The listing builds one solid part. Answer for the finished solid, in the listing's coordinates (mm). A direction names the side the tool comes from. Give positions to 0.01 mm unless a question says otherwise; leave off trailing zeros. Order: outer loops, then holes, each group sorted by start corner. A loop starts at its lowest first (then second) coordinate and runs counter-clockwise, first axis right, second up. Notation, with made-up numbers: (-4, 20) - (26, 20) arc R33 cw to (26, 54) - close; hole circle Ø6 at (79.25, -31.75). An arc over 180 degrees is marked (long way). Answer as a JSON object with one key per item and string values. Group by question number.
Q1. For faces 1 (the face through (91, 11, -11.5)), 2 (the face through (167.3, 15.2, -10)), 3 (the face through (151.831, 5.526, -13.021)), determine the directions among +Z, -Z, +X, -X, +Y, -Y from which every point of the face is accessible in a straight line to the end or side of a thin tool.
Q2. Consider line 1 (X direction, y = 13.25, z = 0); line 2 (X direction, y = 19, z = 5.5); line 3 (Y direction, x = 26.5, z = -13.25). Determine where each line is inside the solid, lowest interval first.
Q3. A cutting plane is placed at C-C, the plane y = 5. Give the vertices of the cut face in (x, z).
Q4. Given pin 1 (5.5 mm diameter, centred on x = 26.5, y = 5, fed in from +Z); pin 2 (4 mm diameter, centred on y = 13.5, z = 11, fed in from -X); pin 3 (8 mm diameter, centred on y = 9, z = 0.5, fed in from +X); pin 4 (1 mm diameter, centred on y = 13.5, z = 8, fed in from -X), each flat-ended and moving along its own axis, determine where each tip first touches the part or whether it passes through.
Q5. A cutting plane is placed at A-A, the plane x = 26.5. Give the vertices of the cut face in (y, z).
Q6. A cutting plane is placed at B-B, the plane z = 0. Give the vertices of the cut face in (x, y).
Q7. A cutting plane is placed at D-D, the plane y = 20.5. Count the separate pieces of the cut face and the enclosed holes in it, and give its area (3 significant figures).
Q8. The mould has two halves that part along Z. Classify faces 4 (the face through (98, 0, -12)), 5 (the face through (189.7, 14.79, 6.18)), 6 (the face through (89, 11, -14.5)), 7 (the face through (12.7, 15.2, -10)): released by +Z, released by -Z, zero draft, split by the parting line, or undercut.
from build123d import *

# Parameters (mm, degrees)
SKETCH1_R           = 11.5
BOSS_EXTRUDE1_DEPTH = 30
FILLET1_R           = 3
SKETCH2_R           = 70
SKETCH2_R_2         = 1.75
CUT_EXTRUDE1_DEPTH  = 30
FILLET2_R           = 3


with BuildPart() as part:
    # Sketch1 → Boss-Extrude1 (new body)
    with BuildSketch(Plane(origin=(0, 0, 0), x_dir=(1, 0, 0), z_dir=(0, 1, 0))):
        with BuildLine():
            Line((0, 14.5), (180, 14.5))
            ThreePointArc((180, 14.5), (184.663689527, -13.729530218), (171.168239134, 11.5))
            Line((171.168239134, 11.5), (8.831760866, 11.5))
            ThreePointArc((8.831760866, 11.5), (-4.663689527, -13.729530218), (0, 14.5))
        make_face()
        with Locations(Location((0, 0, 0), (0, 0, 270))):
            Circle(SKETCH1_R, mode=Mode.SUBTRACT)
        with Locations(Location((180, 0, 0), (0, 0, 270))):
            Circle(SKETCH1_R, mode=Mode.SUBTRACT)
    extrude(amount=BOSS_EXTRUDE1_DEPTH)

    # Fillet1
    fillet1_edges = [part.edges().sort_by_distance(p)[0] for p in [
        (171.168239134, 15, -11.5),
        (8.831760866, 15, -11.5),
    ]]
    fillet(fillet1_edges, radius=FILLET1_R)

    # Sketch2 → Cut-Extrude1 (cut)
    with BuildSketch(Plane(origin=(0, 0, -14.5), x_dir=(-1, 0, 0), z_dir=(0, 0, -1))):
        with Locations((-90, 85.31324406)):
            Circle(SKETCH2_R)
        with Locations((-26.5, 5)):
            Circle(SKETCH2_R_2)
        with Locations((-153.5, 5)):
            Circle(SKETCH2_R_2)
    extrude(amount=-CUT_EXTRUDE1_DEPTH, mode=Mode.SUBTRACT)

    # Fillet2
    fillet2_edges = [part.edges().sort_by_distance(p)[0] for p in [
        (90, 15.31324406, -14.5),
    ]]
    fillet(fillet2_edges, radius=FILLET2_R - 0.0001)  # a hair under: the kernel refuses the full size


solid = part.part
Reply:
{
 "1": {"face 1": "+Z, +Y, -Y", "face 2": "+Y, -Y", "face 3": "+Z, -Z"},
 "2": {"line 1": "x = -14.5 to -11.5, 11.5 to 14.5, 165.5 to 168.5, 191.5 to 194.5", "line 2": "x = -13.42 to -10.1, 10.1 to 13.42, 166.58 to 169.9, 190.1 to 193.42", "line 3": "y = 0 to 3.25, 6.75 to 30"},
 "3": {"outline": "(0, -14.5) - (24.75, -14.5) - (24.75, -11.5) - (15.3, -11.5) arc R3 cw to (12.67, -7.04) arc R14.5 ccw (long way) to start; (28.25, -14.5) - (151.75, -14.5) - (151.75, -11.5) - (28.25, -11.5) - close; (155.25, -14.5) - (180, -14.5) arc R14.5 ccw (long way) to (167.33, -7.04) arc R3 cw to (164.7, -11.5) - (155.25, -11.5) - close; hole circle Ø23 at (0, 0); hole circle Ø23 at (180, 0)"},
 "4": {"pin 1": "stops at z = -11.5", "pin 2": "stops at x = -11.37", "pin 3": "stops at x = 194.5", "pin 4": "stops at x = -12.41"},
 "5": {"outline": "(0, -14.5) - (3.25, -14.5) - (3.25, -11.5) - (0, -11.5) - close; (6.75, -14.5) - (30, -14.5) - (30, -11.5) - (6.75, -11.5) - close"},
 "6": {"outline": "(-14.5, 0) - (-11.5, 0) - (-11.5, 30) - (-14.5, 30) - close; (11.5, 0) - (14.5, 0) - (14.5, 30) - (11.5, 30) - close; (165.5, 0) - (168.5, 0) - (168.5, 30) - (165.5, 30) - close; (191.5, 0) - (194.5, 0) - (194.5, 30) - (191.5, 30) - close"},
 "7": {"separate pieces": "2", "enclosed holes": "2", "area": "841 mm^2"},
 "8": {"face 4": "zero draft", "face 5": "undercut", "face 6": "released by -Z", "face 7": "undercut"}
}
